Check sheet for the modelled part. Datum: model origin and axes. Units: mm. Face numbers are marked on the shaded views. A direction names the side the tool comes from. Give positions to 0.01 mm unless a question says otherwise; leave off trailing zeros. Loops run counter-clockwise (first coordinate to the right, second up) from the corner with the lowest first, then second, coordinate; pieces in that order, holes last. Notation, with made-up numbers: (55, 69.5) -> (103, 69.5) arc R22 ccw to (103, 107.5) -> close; hole circle Ø9 at (13, 71). An arc over 180 degrees is marked (long way). Answer as CSV lines item,"result". Start each with the question number.
(1) Access from +Z, -Z, +X, -X, +Y, -Y to the whole of each face (thin tool, end or side, straight path). Record for the marked faces 1, 2 and 3.
(2) Section check B-B on x = 2.75. Enter the section's corners in (y, z) (3 decimals), plus the area to 3 significant figures.
(3) Material ranges on line 1 (Y direction, x = 1.75, z = -50); line 2 (Y direction, x = 5.25, z = -48.85); line 3 (Z direction, x = 1.5, y = -20), recorded low to high. Write a range as from..to.
(4) Section check C-C on z = -49.5. State how many separate pieces and enclosed holes the cut face has, plus the area to 3 significant figures.
(5) Release check for a two-part mould opening along Y. For the marked faces 4, 5, 6 and 7 record: pulls with the +Y half, pulls with the -Y half, needs draft (parallel to the pull), parting line crosses it, or undercut.
(6) Section check A-A on y = -25. Enter the section's corners in (x, z) (3 decimals), plus the area to 3 significant figures.
(7) Gauge pin test, flat ends, axial feed: pin 1 Ø0.8 at (y, z) = (-22, -45.5) entering from +X; pin 2 Ø8 at (y, z) = (-7, -21) entering from +X; pin 3 Ø3 at (x, z) = (4, -6.5) entering from +Y; pin 4 Ø1.9 at (y, z) = (-25, -48.85) entering from +X. Record the tip position at first contact, or that the pin passes through.
(8) Section check D-D on z = -37.5. Enter the section's corners in (x, y).
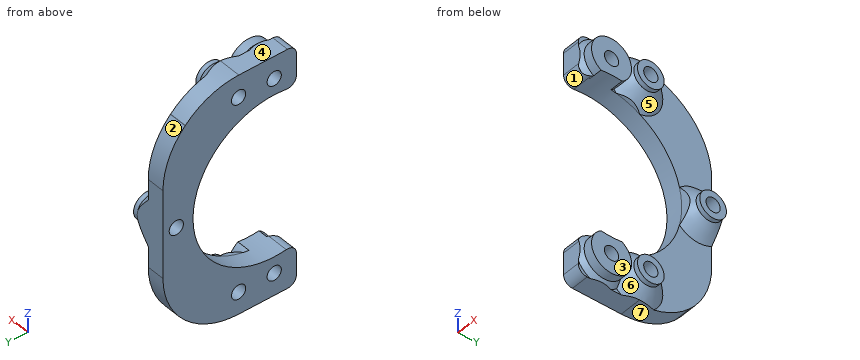
from build123d import *

# Parameters (mm, degrees)
SKETCH_1_W               = 53.85
SKETCH_1_H               = 30
SKETCH_1_R               = 1.6
EXTRUDE_1_DEPTH          = 4
SKETCH_7_R               = 4.5
SKETCH_7_R_2             = 1.6
EXTRUDE_3_DEPTH          = 3
CUT_EXTRUDE_1_DEPTH      = 62.772344136
CUT_EXTRUDE_1_DEPTH_BACK = 4
SKETCH_2_R               = 18.25
CHAMFER_1_SIZE           = 10
SKETCH_3_R               = 3
EXTRUDE_2_DEPTH          = 4
SKETCH_4_R               = 1.6
CUT_EXTRUDE_2_DEPTH      = 63.159653313
CHAMFER_3_SIZE           = 3
CHAMFER_4_SIZE           = 1
FILLET_1_R               = 2
FILLET_2_R               = 17


with BuildPart() as part:
    # 草图1 → 凸台-拉伸1 (new body)
    with BuildSketch(Plane(origin=(0, 0, 0), x_dir=(0, 0, -1), z_dir=(1, 0, 0))):
        with Locations((26.925, -15)):
            Rectangle(SKETCH_1_W, SKETCH_1_H)
        with Locations((5, -25)):
            Circle(SKETCH_1_R, mode=Mode.SUBTRACT)
        with Locations((48.85, -25)):
            Circle(SKETCH_1_R, mode=Mode.SUBTRACT)
    extrude(amount=EXTRUDE_1_DEPTH)

    # 草图7 → 凸台-拉伸3 (add)
    # profile 1 of 2: a face of its own
    with BuildSketch(Plane(origin=(4, 0, 0), x_dir=(0, 0, -1), z_dir=(1, 0, 0))):
        with Locations((5, -25)):
            Circle(SKETCH_7_R)
        with Locations((5, -25)):
            Circle(SKETCH_7_R_2, mode=Mode.SUBTRACT)
    # profile 2 of 2: a face of its own
    with BuildSketch(Plane(origin=(4, 0, 0), x_dir=(0, 0, -1), z_dir=(1, 0, 0))):
        with Locations((48.85, -25)):
            Circle(SKETCH_7_R)
        with Locations((48.85, -25)):
            Circle(SKETCH_7_R_2, mode=Mode.SUBTRACT)
    extrude(amount=EXTRUDE_3_DEPTH)

    # 草图2 → 切除-拉伸1 (cut, two sides: drawn at the far end of the back side and taken through both)
    with BuildSketch(Plane(origin=(4, 0, 0), x_dir=(0, 0, -1), z_dir=(1, 0, 0)).offset(-CUT_EXTRUDE_1_DEPTH_BACK)):
        with Locations((26.925, -25)):
            Circle(SKETCH_2_R)
    extrude(amount=CUT_EXTRUDE_1_DEPTH + CUT_EXTRUDE_1_DEPTH_BACK, mode=Mode.SUBTRACT)

    # 倒角1
    chamfer_1_edges = [part.edges().sort_by_distance(p)[0] for p in [
        (2, 0, 0),
        (2, 0, -53.85),
    ]]
    chamfer(chamfer_1_edges, length=CHAMFER_1_SIZE)

    # 草图3 → 凸台-拉伸2 (add)
    with BuildSketch(Plane(origin=(4, 0, 0), x_dir=(0, 0, -1), z_dir=(1, 0, 0))):
        with Locations((5, -17)):
            Circle(SKETCH_3_R)
        with Locations((48.85, -17)):
            Circle(SKETCH_3_R)
        with Locations(Location((26.925, -3, 0), (0, 0, 90))):
            Circle(SKETCH_3_R)
    extrude(amount=EXTRUDE_2_DEPTH)

    # 草图4 → 切除-拉伸2 (cut, through all)
    with BuildSketch(Plane(origin=(8, 0, 0), x_dir=(0, 0, -1), z_dir=(1, 0, 0))):
        with Locations((5, -17)):
            Circle(SKETCH_4_R)
        with Locations((48.85, -17)):
            Circle(SKETCH_4_R)
        with Locations((26.925, -3)):
            Circle(SKETCH_4_R)
    extrude(amount=-CUT_EXTRUDE_2_DEPTH, mode=Mode.SUBTRACT)

    # 倒角3
    # the kernel refuses this chamfer: 3 mm, written as the material it adds along each edge
    with BuildSketch(Plane(origin=(4, -17, -5), x_dir=(0, 0, -1), z_dir=(0, -1, 0))) as chamfer_3_piece_1_section:
        Polygon((3 + CHAMFER_3_SIZE, 0), (3, CHAMFER_3_SIZE), (3, 0), align=None)
    chamfer_3_piece_1 = revolve(axis=Axis((4, -17, -5), (1, 0, 0)), mode=Mode.PRIVATE)
    chamfer_3_piece_1 = split(chamfer_3_piece_1, bisect_by=Plane(origin=(5.467307701, -17, 0), z_dir=(0, 0, -1)), keep=Keep.TOP, mode=Mode.PRIVATE)
    chamfer_3_piece_1 = chamfer_3_piece_1 - Plane(origin=(5.467307701, -25, -26.925), x_dir=(0, 0, -1), z_dir=(1, 0, 0)) * Cylinder(18.25, 25, mode=Mode.PRIVATE)
    with BuildSketch(Plane(origin=(4, -17, -48.85), x_dir=(0, 0, -1), z_dir=(0, -1, 0))) as chamfer_3_piece_2_section:
        Polygon((3 + CHAMFER_3_SIZE, 0), (3, CHAMFER_3_SIZE), (3, 0), align=None)
    chamfer_3_piece_2 = revolve(axis=Axis((4, -17, -48.85), (1, 0, 0)), mode=Mode.PRIVATE)
    chamfer_3_piece_2 = chamfer_3_piece_2 - Plane(origin=(5.467307729, -25, -26.925), x_dir=(0, 0, -1), z_dir=(1, 0, 0)) * Cylinder(18.25, 24, mode=Mode.PRIVATE)
    chamfer_3_piece_2 = split(chamfer_3_piece_2, bisect_by=Plane(origin=(5.467307729, -17, -53.85), z_dir=(0, 0, 1)), keep=Keep.TOP, mode=Mode.PRIVATE)
    with BuildSketch(Plane(origin=(4, -3, -26.925), x_dir=(0, 1, 0), z_dir=(0, 0, -1))) as chamfer_3_piece_3_section:
        Polygon((3 + CHAMFER_3_SIZE, 0), (3, CHAMFER_3_SIZE), (3, 0), align=None)
    chamfer_3_piece_3 = revolve(axis=Axis((4, -3, -26.925), (1, 0, 0)), mode=Mode.PRIVATE)
    chamfer_3_piece_3 = split(chamfer_3_piece_3, bisect_by=Plane(origin=(4.469931391, 0, -22.187900458), z_dir=(0, -1, 0)), keep=Keep.TOP, mode=Mode.PRIVATE)
    chamfer_3_piece_3 = chamfer_3_piece_3 - Plane(origin=(4.469931391, -25, -26.925), x_dir=(0, 0, -1), z_dir=(1, 0, 0)) * Cylinder(18.25, 24, mode=Mode.PRIVATE)
    add([chamfer_3_piece_1, chamfer_3_piece_2, chamfer_3_piece_3])

    # 倒角4
    # the kernel refuses this chamfer: 1 mm, written as the material it adds along each edge
    with BuildSketch(Plane(origin=(4, -25, -48.85), x_dir=(0, 0.9653833924151701, -0.26083501614809607), z_dir=(0, 0.26083501614809607, 0.9653833924151701))) as chamfer_4_piece_1_section:
        Polygon((4.5, -CHAMFER_4_SIZE), (4.5 + CHAMFER_4_SIZE, 0), (4.5, 0), align=None)
    chamfer_4_piece_1 = revolve(axis=Axis((4, -25, -48.85), (-1, 0, 0)), revolution_arc=255.986755494, mode=Mode.PRIVATE)
    chamfer_4_piece_1 = chamfer_4_piece_1 - Plane(origin=(4.294296116, -25, -26.925), x_dir=(0, 0, -1), z_dir=(1, 0, 0)) * Cylinder(18.25, 22, mode=Mode.PRIVATE)
    chamfer_4_piece_1 = split(chamfer_4_piece_1, bisect_by=Plane(origin=(4.294296116, -30, -51.249638495), z_dir=(0, 1, 0)), keep=Keep.TOP, mode=Mode.PRIVATE)
    chamfer_4_piece_1 = split(chamfer_4_piece_1, bisect_by=Plane(origin=(4.294296116, -20.838072268, -53.85), z_dir=(0, 0, 1)), keep=Keep.TOP, mode=Mode.PRIVATE)
    add(chamfer_4_piece_1)
    with BuildSketch(Plane(origin=(4, -25, -5), x_dir=(0, 0.9653833924151692, 0.26083501614809945), z_dir=(0, 0.26083501614809945, -0.9653833924151692))) as chamfer_4_piece_2_section:
        Polygon((4.5, CHAMFER_4_SIZE), (4.5 + CHAMFER_4_SIZE, 0), (4.5, 0), align=None)
    chamfer_4_piece_2 = revolve(axis=Axis((4, -25, -5), (1, 0, 0)), revolution_arc=255.986755494, mode=Mode.PRIVATE)
    chamfer_4_piece_2 = chamfer_4_piece_2 - Plane(origin=(4.294296117, -25, -26.925), x_dir=(0, 0, -1), z_dir=(1, 0, 0)) * Cylinder(18.25, 22, mode=Mode.PRIVATE)
    chamfer_4_piece_2 = split(chamfer_4_piece_2, bisect_by=Plane(origin=(4.294296117, -30, -2.600361506), z_dir=(0, 1, 0)), keep=Keep.TOP, mode=Mode.PRIVATE)
    chamfer_4_piece_2 = split(chamfer_4_piece_2, bisect_by=Plane(origin=(4.294296117, -20.838072268, 0), z_dir=(0, 0, -1)), keep=Keep.TOP, mode=Mode.PRIVATE)
    add(chamfer_4_piece_2)

    # 圆角1
    # the kernel refuses this fillet: 2 mm, written as the material it takes off along each edge
    with BuildSketch(Plane(origin=(-6.187088914, -30, -9.373290682), x_dir=(0, 0, 1), z_dir=(1, 0, 0))) as fillet_1_piece_1:
        with BuildLine():
            CenterArc((2.474835566, -2), FILLET_1_R, 90, 98.519624254)
            ThreePointArc((0.496905207, -2.296296296), (0.285443162, -1.140143606), (0, 0))
            Line((0, 0), (2.474835566, 0))
        make_face()
    extrude(amount=16.374177829, mode=Mode.SUBTRACT)
    with BuildSketch(Plane(origin=(-6.187088914, -30, -44.476709318), x_dir=(0, 0.977378218113637, -0.21149898051057317), z_dir=(1, 0, 0))) as fillet_1_piece_2:
        with BuildLine():
            CenterArc((2.478181635, -1.995852414), FILLET_1_R, 93.690586551, 98.519624254)
            Line((0.523425199, -2.418850375), (0, 0))
            ThreePointArc((0, 0), (1.174722463, -0.037846719), (2.349444927, 0))
        make_face()
    extrude(amount=16.374177829, mode=Mode.SUBTRACT)
    with BuildSketch(Plane(origin=(-5, -30, -53.85), x_dir=(0, 0, 1), z_dir=(1, 0, 0)), Plane(origin=(-5, -30, 0), x_dir=(0, 1, 0), z_dir=(1, 0, 0))) as fillet_1_piece_3:
        with BuildLine():
            CenterArc((FILLET_1_R, -FILLET_1_R), FILLET_1_R, 90, 90)
            Line((0, -FILLET_1_R), (0, 0))
            Line((0, 0), (FILLET_1_R, 0))
        make_face()
    extrude(amount=14, mode=Mode.SUBTRACT)

    # 圆角2
    # the kernel refuses this fillet: 17 mm, written as the material it takes off along each edge
    with BuildSketch(Plane(origin=(-17.604076401, -10, -53.85), x_dir=(0, -1, 0), z_dir=(1, 0, 0))) as fillet_2_piece_1:
        with BuildLine():
            CenterArc((FILLET_2_R * 0.414213562373, -FILLET_2_R), FILLET_2_R, 90, 45)
            Line((-FILLET_2_R * 0.292893218813, -FILLET_2_R * 0.292893218813), (0, 0))
            Line((0, 0), (FILLET_2_R * 0.414213562373, 0))
        make_face()
    extrude(amount=39.208152802, mode=Mode.SUBTRACT)
    with BuildSketch(Plane(origin=(-17.604076401, 0, -43.85), x_dir=(0, 0, 1), z_dir=(1, 0, 0)), Plane(origin=(-17.604076401, -10, 0), x_dir=(0, -1, 0), z_dir=(1, 0, 0)), Plane(origin=(-17.604076401, 0, -10), x_dir=(0, -0.7071067811865477, 0.7071067811865474), z_dir=(1, 0, 0))) as fillet_2_piece_2:
        with BuildLine():
            CenterArc((FILLET_2_R * 0.414213562373, FILLET_2_R), FILLET_2_R, 225, 45)
            Line((-FILLET_2_R * 0.292893218813, FILLET_2_R * 0.292893218813), (0, 0))
            Line((0, 0), (FILLET_2_R * 0.414213562373, 0))
        make_face()
    extrude(amount=39.208152802, mode=Mode.SUBTRACT)


solid = part.part
Working result:
1,face 1,"+X, -X"
1,face 2,"+Z, +X, -X, +Y"
1,face 3,"+Z, -Z, +X, -Y"
2,outline,"(-30, -51.85) arc R2 ccw to (-28, -53.85) -> (-17.042, -53.85) arc R17 ccw to (-5.021, -48.871) -> (-4.979, -48.829) arc R17 ccw to (0, -36.808) -> (0, -17.042) arc R17 ccw to (-4.979, -5.021) -> (-5.021, -4.979) arc R17 ccw to (-17.042, 0) -> (-28, 0) arc R2 ccw to (-30, -2) -> (-30, -6.898) arc R2 ccw to (-27.704, -8.876) arc R18.25 cw (long way) to (-27.704, -44.974) arc R2 ccw to (-30, -46.952) -> close; hole circle Ø3.2 at (-25, -48.85); hole circle Ø3.2 at (-25, -5); hole circle Ø3.2 at (-17, -48.85); hole circle Ø3.2 at (-17, -5); hole circle Ø3.2 at (-3, -26.925)"
2,area,"743 mm^2"
3,line 1,"y = -30..-26.11, -23.89..-18.11, -15.89..-6.27"
3,line 2,"y = -29.5..-26.6, -23.4..-18.6, -15.4..-12.25"
3,line 3,"z = -53.85..-44.48, -9.37..0"
4,separate pieces,"3"
4,enclosed holes,"0"
4,area,"110 mm^2"
5,face 4,"needs draft"
5,face 5,"undercut"
5,face 6,"undercut"
5,face 7,"pulls with the +Y half"
6,outline,"(0, -53.85) -> (4.5, -53.85) -> (5, -53.35) -> (7, -53.35) -> (7, -50.45) -> (0, -50.45) -> close; (0, -47.25) -> (7, -47.25) -> (7, -45.175) -> (0, -45.175) -> close; (0, -8.675) -> (7, -8.675) -> (7, -6.6) -> (0, -6.6) -> close; (0, -3.4) -> (7, -3.4) -> (7, -0.5) -> (5, -0.5) -> (4.5, 0) -> (0, 0) -> close"
6,area,"74.4 mm^2"
7,pin 1,"stops at x = 7"
7,pin 2,"stops at x = 6.85"
7,pin 3,"stops at y = -2.6"
7,pin 4,"passes through"
8,outline,"(0, -10.13) -> (4, -10.13) -> (4, -0.01) -> (0, -0.01) -> close"
